Input: part model. Units: mm. Frame: model coordinates. Face numbers are marked on the shaded views. A direction names the side the tool comes from. Coordinates: 2 decimals unless noted, no trailing zeros. Loops run counter-clockwise (first coordinate to the right, second up) from the corner with the lowest first, then second, coordinate; pieces in that order, holes last. Notation, with made-up numbers: (55, -22) -> (87, -22) arc R12 ccw to (87, -4) -> close; hole circle Ø6 at (81, -15). An arc over 180 degrees is marked (long way). Put each result on its own line as item: value. Start each with the question number.
1) Contact query for flat-ended pins moving along their axis: P1, Ø4, axis at x = 43, y = 13.5, coming from the -Z side; P2, Ø1.3, axis at y = 12, z = 10.5, coming from the -X side; P3, Ø0.8, axis at x = -38, z = 0.5, coming from the +Y side. Output: stop coordinate, or through.
2) Cut plane C-C (x = -32.5). Return the cut outline in (y, z), plus the area to 3 significant figures.
3) Cut plane B-B (z = 13). Return the cut outline in (x, y), plus the area to 3 significant figures.
4) Cut plane D-D (y = -27.5). Return the cut outline in (x, z).
5) Cut plane A-A (z = 2.25). Return the cut outline in (x, y) (3 decimals), plus the area to 3 significant figures.
6) Set-up query: the marked faces 1, 2 and 3. Return all of +Z, -Z, +X, -X, +Y, -Y with unobstructed straight access to the full face (end or side cutting, diameter ignored); none if empty.
7) Material intervals for L1, parallel to Y at x = -14.5, z = 13.75; L2, parallel to Z at x = -3.5, y = 9; L3, parallel to Y at x = 38, z = 1.5, sorted ascending.
from build123d import *

# Parameters (mm, degrees)
F0_R      = 1.524
F1_DEPTH  = 1.016
F2_W      = 3.5052
F2_H      = 8.9408
F3_DEPTH  = 10.9474
F2_W_2    = 9.906
F4_DEPTH  = 10.9474
F5_R      = 4.445
F6_R      = 0.635
F7_R      = 3.0734
F8_DEPTH  = 10.16
F9_W      = 58.293
F9_H      = 15.2908
F10_DEPTH = 13.081
F11_W     = 15.24
F11_H     = 15.2908
F12_DEPTH = 13.081


with BuildPart() as f1:
    # F0 (on Top) → F1 (new body)
    with BuildSketch(Plane.XY):
        with BuildLine():
            Line((-39.0144, -30.6578), (39.0144, -30.6578))
            ThreePointArc((39.0144, -30.6578), (39.9124256121, -30.2858256121), (40.2844, -29.3878))
            Line((40.2844, -29.3878), (40.2844, 28.4988))
            Line((40.2844, 28.4988), (34.5694, 28.4988))
            Line((34.5694, 28.4988), (34.5694, 30.6578))
            Line((34.5694, 30.6578), (-34.5694, 30.6578))
            Line((-34.5694, 30.6578), (-34.5694, 28.4988))
            Line((-34.5694, 28.4988), (-40.2844, 28.4988))
            Line((-40.2844, 28.4988), (-40.2844, -29.3878))
            ThreePointArc((-40.2844, -29.3878), (-39.9124256121, -30.2858256121), (-39.0144, -30.6578))
        make_face()
        with Locations((-35.2044, 0.1778)):
            Circle(F0_R, mode=Mode.SUBTRACT)
        with Locations((35.2044, 0.1778)):
            Circle(F0_R, mode=Mode.SUBTRACT)
    extrude(amount=F1_DEPTH)

    # F9 (on face) → F10 (join)
    with BuildSketch(Plane.XY.offset(1.016)):
        with Locations((7.4549, -25.6296345744)):
            Rectangle(F9_W, F9_H)
    extrude(amount=F10_DEPTH)



with BuildPart() as f3:
    # F2 (on face) → F3 (new body)
    with BuildSketch(Plane.XY.offset(1.016)):
        with Locations((42.037, 13.3931720629)):
            Rectangle(F2_W, F2_H)
    extrude(amount=F3_DEPTH)

    # F6
    f6_edges = [f3.edges().sort_by_distance(p)[0] for p in [
        (42.037, 8.922772, 11.9634),
        (43.7896, 13.393172, 11.9634),
        (42.037, 17.863572, 11.9634),
        (43.7896, 8.922772, 6.4897),
        (43.7896, 17.863572, 6.4897),
    ]]
    fillet(f6_edges, radius=F6_R)


with BuildPart() as f4:
    # F2 (on face) → F4 (new body)
    with BuildSketch(Plane.XY.offset(1.016)):
        with Locations((35.3314, 13.3931720629)):
            Rectangle(F2_W_2, F2_H)
    extrude(amount=F4_DEPTH)

    # F5
    f5_edges = [f4.edges().sort_by_distance(p)[0] for p in [
        (35.3314, 8.922772, 11.9634),
        (35.3314, 17.863572, 11.9634),
    ]]
    fillet(f5_edges, radius=F5_R)


with BuildPart() as f8_tool:
    # F7 (on face) → F8 (new body)
    with BuildSketch(Plane.YZ.offset(43.7896)):
        with Locations((13.3931720629, 7.5184)):
            Circle(F7_R)
    extrude(amount=-F8_DEPTH)


with BuildPart() as f3_1:
    add(f3.part)

    # F8: cut by f8_tool
    add(f8_tool.part, mode=Mode.SUBTRACT)


with BuildPart() as f4_1:
    add(f4.part)

    # F8: cut by f8_tool
    add(f8_tool.part, mode=Mode.SUBTRACT)


with BuildPart() as f1_1:
    add(f1.part)

    add(f3_1.part)  # F12 merges F3

    add(f4_1.part)  # F12 merges F4
    # F11 (on face) → F12 (join)
    with BuildSketch(Plane.XY.offset(1.016)):
        with Locations((-29.4894, -25.6296345744)):
            Rectangle(F11_W, F11_H)
    extrude(amount=F12_DEPTH)


solid = f1_1.part
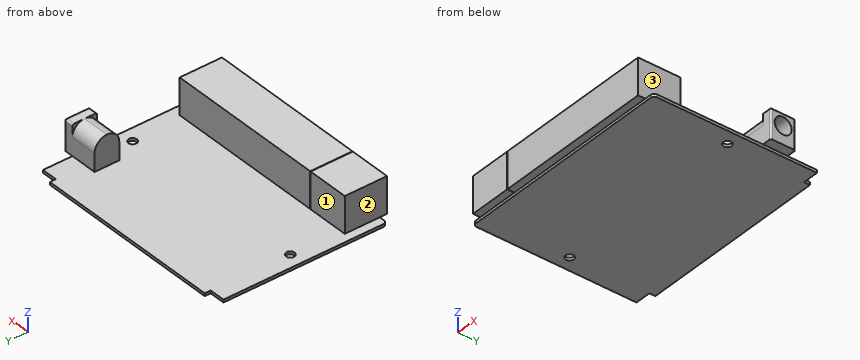
Results found:
1. P1: stops at z = 1.02
1. P2: stops at x = 30.38
1. P3: stops at y = 28.5
2. outline: (-33.28, 1.02) -> (-30.66, 1.02) -> (-30.66, 0) -> (30.66, 0) -> (30.66, 1.02) -> (-17.98, 1.02) -> (-17.98, 14.1) -> (-33.28, 14.1) -> close
2. area: 262 mm2
3. outline: (-37.11, -33.28) -> (-21.87, -33.28) -> (-21.87, -17.98) -> (-37.11, -17.98) -> close; (-21.69, -33.28) -> (36.6, -33.28) -> (36.6, -17.98) -> (-21.69, -17.98) -> close
3. area: 1,120 mm2
4. outline: (-40.28, 0) -> (40.28, 0) -> (40.28, 1.02) -> (36.6, 1.02) -> (36.6, 14.1) -> (-21.69, 14.1) -> (-21.69, 1.02) -> (-21.87, 1.02) -> (-21.87, 14.1) -> (-37.11, 14.1) -> (-37.11, 1.02) -> (-40.28, 1.02) -> close
5. outline: (-37.109, -33.275) -> (-21.869, -33.275) -> (-21.869, -17.984) -> (-37.109, -17.984) -> close; (-21.692, -33.275) -> (36.601, -33.275) -> (36.601, -17.984) -> (-21.692, -17.984) -> close; (30.378, 8.923) -> (43.155, 8.923) arc R0.635 ccw to (43.79, 9.558) -> (43.79, 17.229) arc R0.635 ccw to (43.155, 17.864) -> (30.378, 17.864) -> close
5. area: 1,240 mm2
6. face 1: +Z, +X, -X, +Y
6. face 2: +Z, -X, +Y, -Y
6. face 3: +Z, +X, -Y
7. L1: y = -33.28 to -17.98
7. L2: z = 0 to 1.02
7. L3: y = 8.92 to 17.86
